from build123d import *

# Parameters (mm, degrees)
F0_W     = 42.3
F0_H     = 42.3
F0_R     = 1.5
F1_DEPTH = 22
F2_R     = 2.5
F3_DEPTH = 16
F4_SIZE  = 4


with BuildPart() as f1:
    # F0 (on Front) → F1 (new body)
    with BuildSketch(Plane.XZ):
        Rectangle(F0_W, F0_H)
        with Locations((-15.5, -15.5)):
            Circle(F0_R, mode=Mode.SUBTRACT)
        with Locations((15.5, -15.5)):
            Circle(F0_R, mode=Mode.SUBTRACT)
        with Locations((-15.5, 15.5)):
            Circle(F0_R, mode=Mode.SUBTRACT)
        with Locations((15.5, 15.5)):
            Circle(F0_R, mode=Mode.SUBTRACT)
    extrude(amount=F1_DEPTH)

    # F2 (on face) → F3 (join)
    with BuildSketch(Plane.XZ.offset(22)):
        Circle(F2_R)
    extrude(amount=F3_DEPTH)

    # F4
    f4_edges = [f1.edges().sort_by_distance(p)[0] for p in [
        (21.15, -11, 21.15),
        (21.15, -11, -21.15),
        (-21.15, -11, 21.15),
        (-21.15, -11, -21.15),
    ]]
    chamfer(f4_edges, length=F4_SIZE)


solid = f1.part
Input: part model. Units: mm. Frame: model coordinates. A direction names the side the tool comes from. Coordinates: 2 decimals unless noted, no trailing zeros. Write each loop counter-clockwise with the first axis right and the second up, starting at its lowest first coordinate (ties: lowest second). Pieces come first, ordered by that corner, then holes. Notation, with made-up numbers: M 48.25,-31 L 105.25,-31 A22 cw 105.25,-8 Z; hole C 14.5,-36.75 d5. An arc over 180 degrees is marked long. Answer as a JSON object with one key per item and string values. Group by question number.
(1) Set-up query: faces 1 (the face through (-0.54, -29.89, -2.44)), 2 (the face through (0, -38, 0)). Return all of +Z, -Z, +X, -X, +Y, -Y with unobstructed straight access to the full face (end or side cutting, diameter ignored); none if empty.
(2) Ray query, line 1 along Z through (x, y) = (15.5, -13.75); line 2 along Y through (x, z) = (-18.5, -13); line 3 along X through (y, z) = (-14, 15). Return the intervals inside material, ascending. Write a range as [from, to].
(3) Section A-A on x = -15.5. Output: boundary loops of the cut face in (y, z), plus the area to 3 significant figures.
(4) Section C-C on y = -5.5. Output: boundary loops of the cut face in (x, z).
(5) Section B-B on z = 15.5. Output: boundary loops of the cut face in (x, y), plus the area to 3 significant figures.
(6) Section D-D on x = 0. Output: boundary loops of the cut face in (y, z).
(7) Mould query, pull axis X, two halves, no side actions, for faces 3 (the face through (-5, -22, 0)), 4 (the face through (21.15, -11, 0)), 5 (the face through (-17, -10.85, -15.43)), 6 (the face through (-17, -10.85, 15.57)). Classes: pulls with the +X half, pulls with the -X half, needs draft (parallel to the pull), parting line crosses it, or undercut.
(8) Contact query for flat-ended pins moving along their axis: P1, Ø12, axis at x = 7.5, z = 9.5, coming from the +Y side; P2, Ø5, axis at x = -6.5, z = 3.5, coming from the -Y side. Output: stop coordinate, or through.
Result set:
{
 "1": {"face 1": "-Y", "face 2": "+Z, -Z, +X, -X, -Y"},
 "2": {"line 1": "z = [-21.15, -17], [-14, 14], [17, 21.15]", "line 2": "y = [-22, 0]", "line 3": "x = [-21.15, -16.91], [-14.09, 14.09], [16.91, 21.15]"},
 "3": {"outline": "M -22,-21.15 L 0,-21.15 L 0,-17 L -22,-17 Z; M -22,-14 L 0,-14 L 0,14 L -22,14 Z; M -22,17 L 0,17 L 0,21.15 L -22,21.15 Z", "area": "799 mm2"},
 "4": {"outline": "M -21.15,-17.15 L -17.15,-21.15 L 17.15,-21.15 L 21.15,-17.15 L 21.15,17.15 L 17.15,21.15 L -17.15,21.15 L -21.15,17.15 Z; hole C -15.5,-15.5 d3; hole C -15.5,15.5 d3; hole C 15.5,-15.5 d3; hole C 15.5,15.5 d3"},
 "5": {"outline": "M -21.15,-22 L -17,-22 L -17,0 L -21.15,0 Z; M -14,-22 L 14,-22 L 14,0 L -14,0 Z; M 17,-22 L 21.15,-22 L 21.15,0 L 17,0 Z", "area": "799 mm2"},
 "6": {"outline": "M -38,-2.5 L -22,-2.5 L -22,-21.15 L 0,-21.15 L 0,21.15 L -22,21.15 L -22,2.5 L -38,2.5 Z"},
 "7": {"face 3": "needs draft", "face 4": "pulls with the +X half", "face 5": "undercut", "face 6": "undercut"},
 "8": {"P1": "stops at y = 0", "P2": "stops at y = -22"}
}
